Check sheet for the drawn part. Datum: minimum x, y, z corner. Units: mm. Coordinates: 2 decimals unless noted, no trailing zeros. Order: outer loops, then holes, each group sorted by start corner. A loop starts at its lowest first (then second) coordinate and runs counter-clockwise, first axis right, second up.
Q1. Draft check along Y on the marked faces 1, 2 and 3. Enter one of: pulls with the +Y half, pulls with the -Y half, needs draft (parallel to the pull), parting line crosses it, or undercut.
Q2. Depth check by flat-ended pin: P1, Ø1.5, axis at x = 13.5, z = 2, coming from the -Y side. Enter the tip coordinate at first touch or a pass-through.
Q3. Cross-section at C-C, the plane x = 2.25. Record the boundary of the cut face in (y, z) (1 decimal).
Q4. Cross-section at A-A, the plane y = 3.5. Record the boundary of the cut face in (x, z) (1 decimal).
Q5. Cross-section at D-D, the plane y = 6.25. Record the boundary of the cut face in (x, z) (1 decimal), and give its area (3 significant figures).
Q6. Thickness scan on line 1 (X direction, y = 3.25, z = 3.55); line 2 (X direction, y = 4.75, z = 2.05) (1 decimal); line 3 (Y direction, x = 2.75, z = 4.1). Record the ranges inside material, lowest first.
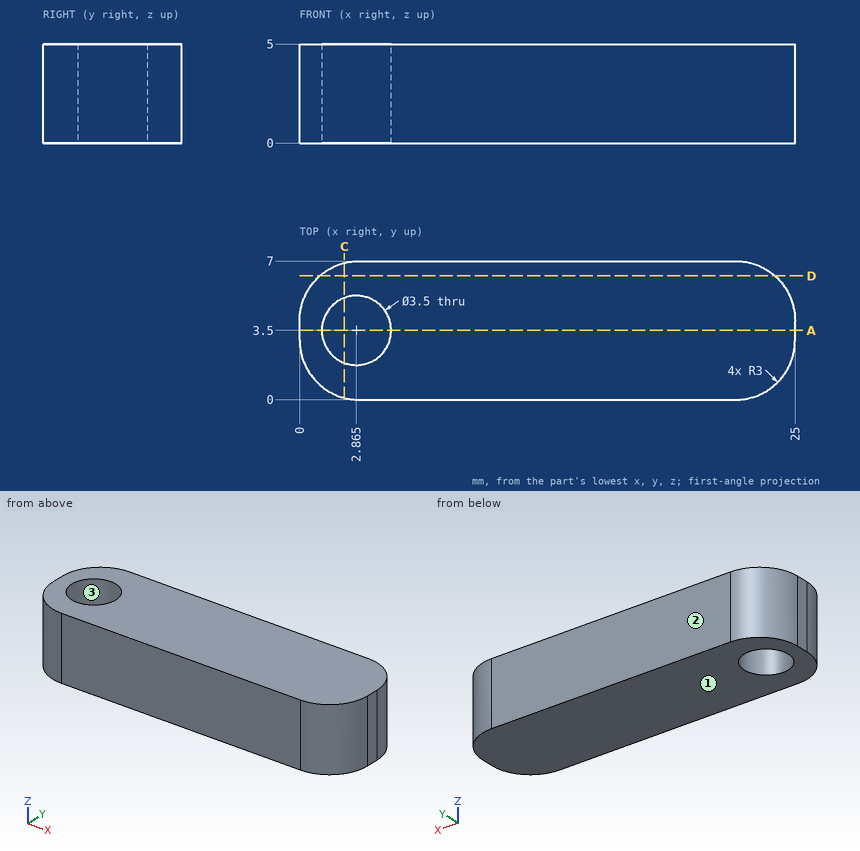
Check values:
1. face 1: needs draft
1. face 2: pulls with the +Y half
1. face 3: undercut
2. P1: stops at y = 0
3. outline: (0.1, 0) - (1.9, 0) - (1.9, 5) - (0.1, 5) - close; (5.1, 0) - (6.9, 0) - (6.9, 5) - (5.1, 5) - close
4. outline: (0, 0) - (1.1, 0) - (1.1, 5) - (0, 5) - close; (4.6, 0) - (25, 0) - (25, 5) - (4.6, 5) - close
5. outline: (1, 0) - (24, 0) - (24, 5) - (1, 5) - close
5. area: 115 mm2
6. line 1: x = 0 to 1.13, 4.6 to 25
6. line 2: x = 0.1 to 1.6, 4.1 to 24.9
6. line 3: y = 0.01 to 1.75, 5.25 to 6.99
